Work out the finished part from the listing and answer in its coordinate system (mm). A direction names the side the tool comes from. Give positions to 0.01 mm unless a question says otherwise; leave off trailing zeros. Order: outer loops, then holes, each group sorted by start corner. A loop starts at its lowest first (then second) coordinate and runs counter-clockwise, first axis right, second up. Notation, with made-up numbers: (-10, 36) -> (3, 36) arc R30 cw to (3, 74) -> close; hole circle Ø6 at (85.25, 40). An arc over 180 degrees is marked (long way). Answer as CSV lines item,"result". Start each with the question number.
1. A cutting plane is placed at A-A (y = 15). Give the vertices of the cut face in (x, z).
2. A cutting plane is placed at C-C (y = -133.5). Give the vertices of the cut face in (x, z), then the cut area to 3 significant figures.
3. A cutting plane is placed at D-D (z = 137). Give the vertices of the cut face in (x, y).
4. For a pull along Y with two mould halves and no side action, classify faces 1 (the cylindrical face through (-100.01, 43.61, -260.28)), 2 (the flat face through (-110, 150, -187)), 3 (the flat face through (-114, -109, 1000)) as released by +Y, released by -Y, zero draft, split by the parting line, or undercut.
5. A cutting plane is placed at B-B (x = -15.5). Give the vertices of the cut face in (y, z).
6. Flat-ended cylindrical pins translate along their axes: pin 1 (2 mm diameter, centred on x = -23.5, z = 49.5, fed in from +Y); pin 2 (10 mm diameter, centred on y = -107.5, z = -246.5, fed in from +X); pin 3 (9 mm diameter, centred on x = 12.5, z = 716.5, fed in from +Y). Find the tip coordinate at first contact, or state that the pin passes through.
7. Find the intervals of material crossed by L1, parallel to Z at x = -88, y = -92; L2, parallel to Z at x = -173, y = 27.5; L3, parallel to X at y = -137.5, z = 663.5, in increasing order.
8. For faces 4 (the flat face through (-114, -180, 493)), 5 (the flat face through (-114, -33, -360)), 6 (the cylindrical face through (-12.38, -134.49, -380.28)), 7 (the flat face through (-110, 126, 20)), 8 (the cylindrical face through (-212.388, -134.489, -379.72)), determine the directions among +Z, -Z, +X, -X, +Y, -Y from which every point of the face is accessible in a straight line to the end or side of a thin tool.
from build123d import *

# Parameters (mm, degrees)
BOSS_EXTRUDE1_DEPTH = 1000
BOSS_EXTRUDE2_DEPTH = 20
SKETCH3_W           = 284.767845469
SKETCH3_H           = 40
BOSS_EXTRUDE4_DEPTH = 400
SKETCH4_W           = 284.767845469
SKETCH4_H           = 40
BOSS_EXTRUDE5_DEPTH = 290
SKETCH7_R           = 12
CUT_EXTRUDE1_DEPTH  = 372
FILLET1_R           = 150


with BuildPart() as part:
    # Sketch1 → Boss-Extrude1 (new body)
    with BuildSketch(Plane.XY):
        with BuildLine():
            Line((-223.996890487, 0), (-253.996890487, 0))
            Line((-253.996890487, 0), (-253.996890487, -180))
            Line((-253.996890487, -180), (30, -180))
            Line((30, -180), (30, 0))
            Line((30, 0), (0, 0))
            ThreePointArc((0, 0), (-111.998445243, -76.914639806), (-223.996890487, 0))
        make_face()
    extrude(amount=BOSS_EXTRUDE1_DEPTH)

    # Sketch2 → Boss-Extrude2 (add)
    with BuildSketch(Plane(origin=(0, 0, 0), x_dir=(-1, 0, 0), z_dir=(0, 0, -1))):
        Polygon((-30, 110), (-30, 0), (0, 0), (0, 110), (223.996890487, 110), (223.996890487, 0), (253.996890487, 0), (254.767845469, 0), (254.767845469, 110), (254.767845469, 150), (223.996890487, 150), (0, 150), (-30, 150), align=None)
    extrude(amount=-BOSS_EXTRUDE2_DEPTH)

    # Sketch3 → Boss-Extrude4 (add)
    with BuildSketch(Plane(origin=(0, 0, 0), x_dir=(-1, 0, 0), z_dir=(0, 0, -1))):
        with Locations((112.383922735, 130)):
            Rectangle(SKETCH3_W, SKETCH3_H)
    extrude(amount=BOSS_EXTRUDE4_DEPTH)

    # Sketch4 → Boss-Extrude5 (add)
    with BuildSketch(Plane.XZ.offset(-110)):
        with Locations((-112.383922735, -380)):
            Rectangle(SKETCH4_W, SKETCH4_H)
        with Locations((-112.383922735, -260)):
            Rectangle(SKETCH4_W, SKETCH4_H)
    extrude(amount=BOSS_EXTRUDE5_DEPTH)

    # Sketch7 → Cut-Extrude1 (cut)
    with BuildSketch(Plane(origin=(0, 0, -400), x_dir=(-1, 0, 0), z_dir=(0, 0, -1))):
        with Locations((111.998445243, 43.085360194)):
            Circle(SKETCH7_R)
    extrude(amount=-CUT_EXTRUDE1_DEPTH, mode=Mode.SUBTRACT)

    # Fillet1
    # the kernel refuses this fillet: 150 mm, written as the material it takes off along each edge
    with BuildSketch(Plane(origin=(-254.767845469, -180, 15), x_dir=(0, 1, 0), z_dir=(0, 0, -1))) as fillet1_piece_1_section:
        with BuildLine():
            CenterArc((FILLET1_R, FILLET1_R), FILLET1_R, 180, 90)
            Line((0, FILLET1_R), (0, 0))
            Line((0, 0), (FILLET1_R, 0))
        make_face()
    fillet1_piece_1 = extrude(amount=790, mode=Mode.PRIVATE)
    fillet1_piece_1 = split(fillet1_piece_1, bisect_by=Plane(origin=(-254.387947187, -110.019667164, -240), z_dir=(0, 0, -1)), keep=Keep.TOP, mode=Mode.PRIVATE)
    add(fillet1_piece_1, mode=Mode.SUBTRACT)
    with BuildSketch(Plane(origin=(30, -180, -775), x_dir=(0, 1, 0), z_dir=(0, 0, 1))) as fillet1_piece_2_section:
        with BuildLine():
            CenterArc((FILLET1_R, FILLET1_R), FILLET1_R, 180, 90)
            Line((0, FILLET1_R), (0, 0))
            Line((0, 0), (FILLET1_R, 0))
        make_face()
    fillet1_piece_2 = extrude(amount=790, mode=Mode.PRIVATE)
    fillet1_piece_2 = split(fillet1_piece_2, bisect_by=Plane(origin=(-3.505190842, -146.494809158, -240), z_dir=(0, 0, -1)), keep=Keep.TOP, mode=Mode.PRIVATE)
    add(fillet1_piece_2, mode=Mode.SUBTRACT)
    with BuildSketch(Plane(origin=(-254.767845469, -180, -655), x_dir=(0, 1, 0), z_dir=(0, 0, 1)), Plane(origin=(30, -180, -240), x_dir=(0, 1, 0), z_dir=(0, 0, -1))) as fillet1_piece_3:
        with BuildLine():
            CenterArc((FILLET1_R, -FILLET1_R), FILLET1_R, 90, 90)
            Line((0, -FILLET1_R), (0, 0))
            Line((0, 0), (FILLET1_R, 0))
        make_face()
    extrude(amount=415, mode=Mode.SUBTRACT)


solid = part.part
Answer sheet:
1,outline,"(-254.77, -400) -> (30, -400) -> (30, -360) -> (-254.77, -360) -> close; (-254.77, -280) -> (30, -280) -> (30, -240) -> (-254.77, -240) -> close; (-254.77, 0) -> (-224, 0) -> (-224, 20) -> (-254.77, 20) -> close; (0, 0) -> (30, 0) -> (30, 20) -> (0, 20) -> close"
2,outline,"(-254, 0) -> (30, 0) -> (30, 1000) -> (-254, 1000) -> close; (-213.34, -400) -> (-11.43, -400) -> (-11.43, -360) -> (-213.34, -360) -> close; (-213.34, -280) -> (-11.43, -280) -> (-11.43, -240) -> (-213.34, -240) -> close"
2,area,"300,000 mm^2"
3,outline,"(-254, -180) -> (30, -180) -> (30, 0) -> (0, 0) arc R120 cw to (-224, 0) -> (-254, 0) -> close"
4,face 1,"undercut"
4,face 2,"released by +Y"
4,face 3,"zero draft"
5,outline,"(-180, 0) -> (-28.25, 0) -> (-28.25, 1000) -> (-180, 1000) -> close; (-137.61, -400) -> (150, -400) -> (150, 20) -> (110, 20) -> (110, -240) -> (-137.61, -240) -> (-137.61, -280) -> (110, -280) -> (110, -360) -> (-137.61, -360) -> close"
6,pin 1,"stops at y = -36.85"
6,pin 2,"stops at x = 11.32"
6,pin 3,"stops at y = 0"
7,L1,"z = -400 to -360, -280 to -240, 0 to 1000"
7,L2,"z = -400 to -360, -280 to -240"
7,L3,"x = -254 to 30"
8,face 4,"+Z, -Z, +X, -X, -Y"
8,face 5,"+X, -X, -Y"
8,face 6,"-Z, +X, -Y"
8,face 7,"+Z, +X, -X, +Y"
8,face 8,"-Z, -X, -Y"
